Can you work these out from the model? Positions are in its coordinate system, mm. A direction names the side the tool comes from. Round coordinates to 2 decimals unless told otherwise and drop trailing zeros. Order: outer loops, then holes, each group sorted by start corner. A loop starts at its lowest first (then second) coordinate and runs counter-clockwise, first axis right, second up.
Q1. We'd pull the mould along Y, two halves only. Please class faces 1 (the face through (0, -10, 42)), 2 (the face through (-1, 0, 60)), 3 (the face through (0, 0, -3)): pulls with the +Y half, pulls with the -Y half, needs draft (parallel to the pull), parting line crosses it, or undercut.
Q2. If we section it at B-B (y = 0): Please give me the cut outline in (x, z), plus the area to 3 significant figures.
Q3. If we section it at A-A (z = 2): Please give me the cut outline in (x, y), plus the area to 3 significant figures.
Q4. For faces 4 (the face through (-5, 0, -5)), 5 (the face through (-100, 0, 55)), 6 (the face through (3, -3, -3)), 7 (the face through (5, -4, -5)), which set-ups out of +Z, -Z, +X, -X, +Y, -Y let a thin tool reach every point of the face, with its end or its side?
Q5. Will these pins go through, and if not, where does the flat tip stop? P1, Ø1, axis at x = 79, y = 1.5, coming from the -Z side; P2, Ø2, axis at y = -5, z = -24, coming from the +X side; P3, Ø12, axis at y = -0.5, z = -23, coming from the -X side.
Q6. If I drill on line 1 (X direction, y = -1.25, z = 28); line 2 (X direction, y = -4.5, z = -28); line 3 (Z direction, x = 76, y = -6), over which ranges is the centre line in solid material (lowest first)?
from build123d import *

# Parameters (mm, degrees)
BACK_START      = -5
SKETCH1_W       = 100
SKETCH1_H       = 20
BACK_DEPTH      = 10
CURVE_START     = -5
CURVE_END_DEPTH = 10
SLOT_START      = 5
SLOT_DEPTH      = 5
FRONT_START     = -100
SKETCH11_W      = 10
SKETCH11_H      = 20
FRONT_DEPTH     = 200


with BuildPart() as part:
    # Sketch1 → Back (new body)
    with BuildSketch(Plane(origin=(0, 0, 0), x_dir=(0, 0, -1), z_dir=(1, 0, 0)).offset(BACK_START)):
        Rectangle(SKETCH1_W, SKETCH1_H)
    extrude(amount=BACK_DEPTH)

    # Sketch5 → Curve End (add)
    with BuildSketch(Plane(origin=(0, 0, 0), x_dir=(0, 0, -1), z_dir=(1, 0, 0)).offset(CURVE_START)):
        with BuildLine():
            ThreePointArc((50, 10), (58.658985764, 0), (50, -10))
            Line((50, -10), (48.569993907, -0.102773996))
            ThreePointArc((48.569993907, -0.102773996), (48.658985764, 0), (48.569993907, 0.102773996))
            Line((48.569993907, 0.102773996), (50, 10))
        make_face()
    extrude(amount=CURVE_END_DEPTH)

    # Sketch7 → Slot (cut)
    with BuildSketch(Plane(origin=(0, 0, 0), x_dir=(0, 0, -1), z_dir=(1, 0, 0)).offset(SLOT_START)):
        with BuildLine():
            Line((-40, 3), (45, 3))
            ThreePointArc((45, 3), (48, 0), (45, -3))
            Line((45, -3), (-40, -3))
            ThreePointArc((-40, -3), (-43, 0), (-40, 3))
        make_face()
    extrude(amount=-SLOT_DEPTH, mode=Mode.SUBTRACT)

    # Sketch11 → Front (add)
    with BuildSketch(Plane(origin=(0, 0, 0), x_dir=(0, 0, -1), z_dir=(1, 0, 0)).offset(FRONT_START)):
        with Locations((-55, 0)):
            Rectangle(SKETCH11_W, SKETCH11_H)
    extrude(amount=FRONT_DEPTH)


solid = part.part
Solution:
1. face 1: pulls with the -Y half
1. face 2: needs draft
1. face 3: undercut
2. outline: (-100, 50) - (-5, 50) - (-5, -58.66) - (5, -58.66) - (5, -48) - (0, -48) - (0, 43) - (5, 43) - (5, 50) - (100, 50) - (100, 60) - (-100, 60) - close
2. area: 2,630 mm2
3. outline: (-5, -10) - (5, -10) - (5, -3) - (0, -3) - (0, 3) - (5, 3) - (5, 10) - (-5, 10) - close
3. area: 170 mm2
4. face 4: -Z, -X, +Y, -Y
4. face 5: +Z, -Z, -X, +Y, -Y
4. face 6: +X
4. face 7: -Z, +X, +Y, -Y
5. P1: stops at z = 50
5. P2: stops at x = 5
5. P3: stops at x = -5
6. line 1: x = -5 to 0
6. line 2: x = -5 to 5
6. line 3: z = 50 to 60
